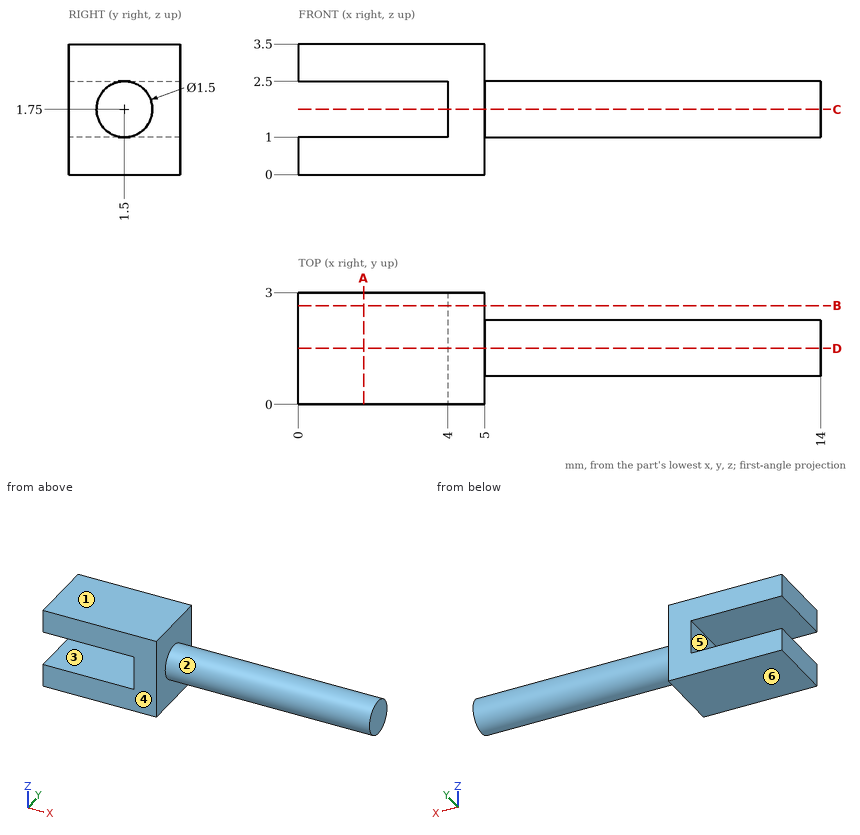
Can you work these out from the drawing? Everything is in mm from the part's minimum corner. A direction names the side the tool comes from. Round coordinates to 2 decimals unless told otherwise and drop trailing zeros. Loops run counter-clockwise (first coordinate to the right, second up) from the corner with the lowest first, then second, coordinate; pieces in that order, holes last. Notation, with made-up numbers: (17.25, -24) - (28.25, -24) arc R21 ccw to (28.25, -3) - close; hole circle Ø9 at (84, 87.5). An arc over 180 degrees is marked (long way). Write item = value, one per line. Start each with the question number.
(1) If we section it at B-B (y = 2.65): Please give me the cut outline in (x, z), and give its area (3 significant figures).
(2) If we section it at C-C (z = 1.75): Please give me the cut outline in (x, y), and give its area (3 significant figures).
(3) If we mould it in two halves opening along Z, with no side actions, what happens to the marked faces 4, 5 and 6? For each: released by +Z, released by -Z, zero draft, split by the parting line, or undercut.
(4) If I drill on probe 1 along Z at (x, y) = (2, 1.45); probe 2 along X at (y, z) = (1, 0.5); probe 3 along X at (y, z) = (0.75, 1.5), over which ranges is the centre line in solid material (lowest first)? Write a range as [from, to].
(5) For the marked faces 1, 2 and 3, which set-ups out of +Z, -Z, +X, -X, +Y, -Y let a thin tool reach every point of the face, with its end or its side?
(6) If we section it at A-A (x = 1.75): Please give me the cut outline in (y, z), and give its area (3 significant figures).
(7) For P1, Ø1.5, axis at x = 8, z = 1, coming from the -Y side; P2, Ø0.8, axis at y = 1.5, z = 2, coming from the -X side, each with a flat end and sliding along its axis, tell me the tip position at first contact or that it passes through.
(8) If we section it at D-D (y = 1.5): Please give me the cut outline in (x, z).
Ans:
q1.outline = (0, 0) - (5, 0) - (5, 3.5) - (0, 3.5) - (0, 2.5) - (4, 2.5) - (4, 1) - (0, 1) - close
q1.area = 11.5 mm²
q2.outline = (4, 0) - (5, 0) - (5, 0.75) - (14, 0.75) - (14, 2.25) - (5, 2.25) - (5, 3) - (4, 3) - close
q2.area = 16.5 mm²
q3.face_4 = zero draft
q3.face_5 = undercut
q3.face_6 = released by -Z
q4.probe_1 = [0, 1], [2.5, 3.5]
q4.probe_2 = [0, 5]
q4.probe_3 = [4, 5]
q5.face_1 = +Z, +X, -X, +Y, -Y
q5.face_2 = +X
q5.face_3 = -X, +Y, -Y
q6.outline = (0, 0) - (3, 0) - (3, 1) - (0, 1) - close; (0, 2.5) - (3, 2.5) - (3, 3.5) - (0, 3.5) - close
q6.area = 6.00 mm²
q7.P1 = 0.75
q7.P2 = 4
q8.outline = (0, 0) - (5, 0) - (5, 1) - (14, 1) - (14, 2.5) - (5, 2.5) - (5, 3.5) - (0, 3.5) - (0, 2.5) - (4, 2.5) - (4, 1) - (0, 1) - close
